Answer from the drawing. Dimensions are ordinates in mm from the lowest x, y and z of the part. A direction names the side the tool comes from. Round coordinates to 2 decimals unless told otherwise and drop trailing zeros. Order: outer loops, then holes, each group sorted by start corner. A loop starts at its lowest first (then second) coordinate and runs counter-clockwise, first axis right, second up.
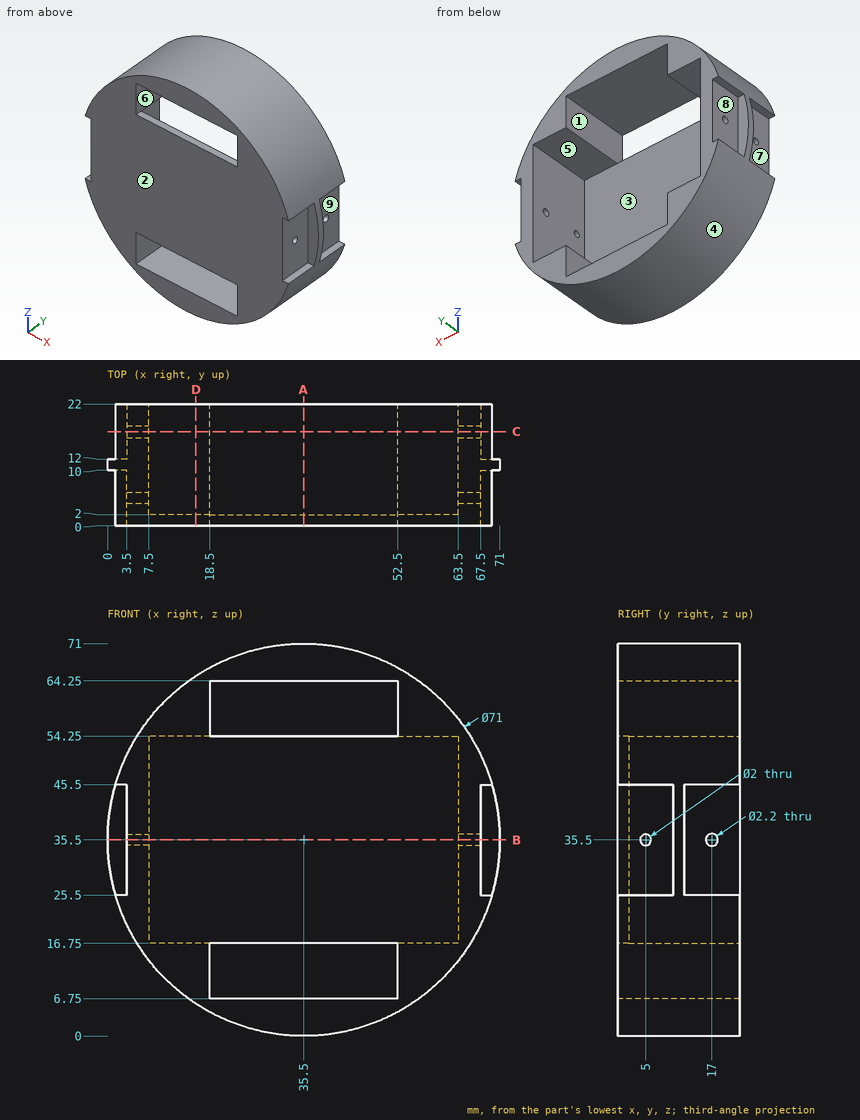
Q1. A cutting plane is placed at C-C, the plane y = 17. Give the vertices of the cut face in (x, z), plus the area to 3 significant figures.
Outcome:
outline: (1.44, 25.5) arc R35.5 ccw to (69.56, 25.5) - (67.5, 25.5) - (67.5, 34.4) - (63.5, 34.4) - (63.5, 16.75) - (52.5, 16.75) - (52.5, 6.75) - (18.5, 6.75) - (18.5, 16.75) - (7.5, 16.75) - (7.5, 34.4) - (3.5, 34.4) - (3.5, 25.5) - close; (1.44, 45.5) - (3.5, 45.5) - (3.5, 36.6) - (7.5, 36.6) - (7.5, 54.25) - (18.5, 54.25) - (18.5, 64.25) - (52.5, 64.25) - (52.5, 54.25) - (63.5, 54.25) - (63.5, 36.6) - (67.5, 36.6) - (67.5, 45.5) - (69.56, 45.5) arc R35.5 ccw to start
area: 1,040 mm2
Q2. A cutting plane is placed at B-B, the plane z = 35.5. Give the number of separate pieces and of enclosed holes in the cut face, plus the area to 3 significant figures.
Outcome:
separate pieces: 5
enclosed holes: 0
area: 268 mm2
Q3. A cutting plane is placed at D-D, the plane x = 16. Give the vertices of the cut face in (y, z).
Outcome:
outline: (0, 5.84) - (22, 5.84) - (22, 16.75) - (2, 16.75) - (2, 54.25) - (22, 54.25) - (22, 65.16) - (0, 65.16) - close
Q4. Flat-ended cylindrical pins translate along their axes: pin 1 (1.6 mm diameter, centred on x = 69, y = 17, fed in from +Z); pin 2 (4 mm diameter, centred on x = 55, z = 43, fed in from +Y); pin 3 (8 mm diameter, centred on x = 53.5, y = 19.5, fed in from +Z). Find the tip coordinate at first contact, or state that the pin passes through.
Outcome:
pin 1: stops at z = 49.32
pin 2: stops at y = 2
pin 3: stops at z = 68.12
Q5. Straight lines are drawn through the part: probe 1 along X at (y, z) = (12.5, 27.5); probe 2 along Y at (x, z) = (4.9, 35.5); probe 3 along Y at (x, z) = (17, 28.5). For each, find the intervals that lie inside material, in ascending order.
Outcome:
probe 1: x = 3.5 to 7.5, 63.5 to 67.5
probe 2: y = 0 to 4, 6 to 15.9, 18.1 to 22
probe 3: y = 0 to 2
Q6. A cutting plane is placed at A-A, the plane x = 35.5. Give the vertices of the cut face in (y, z).
Outcome:
outline: (0, 0) - (22, 0) - (22, 6.75) - (0, 6.75) - close; (0, 16.75) - (2, 16.75) - (2, 54.25) - (0, 54.25) - close; (0, 64.25) - (22, 64.25) - (22, 71) - (0, 71) - close
Q7. For a pull along Z with two mould halves and no side action, classify the marked faces 1, 2, 3 and 4 as released by +Z, released by -Z, zero draft, split by the parting line, or undercut.
Outcome:
face 1: undercut
face 2: zero draft
face 3: undercut
face 4: split by the parting line
Q8. For the marked faces 5, 6, 7, 8 and 9, determine the directions among +Z, -Z, +X, -X, +Y, -Y from which every point of the face is accessible in a straight line to the end or side of a thin tool.
Outcome:
face 5: +Y
face 6: +Y, -Y
face 7: -X, -Y
face 8: -X, +Y
face 9: +X, +Y
